from build123d import *

# Parameters (mm, degrees)
F2_R    = 2
F3_SIZE = 0.75


with BuildPart() as f1:
    # F0 (on Front) → F1 (revolve)
    with BuildSketch(Plane.XZ):
        Polygon((5.5, 0), (6.5, 30), (0, 30), (0, 15), (4, 15), (4, 0), align=None)
    revolve(axis=Axis((0, 0, 0.05881), (0, 0, -1)))

    # F2
    f2_edges = [f1.edges().sort_by_distance(p)[0] for p in [
        (-6.5, 0, 30),
    ]]
    fillet(f2_edges, radius=F2_R)

    # F3
    f3_edges = [f1.edges().sort_by_distance(p)[0] for p in [
        (-5.5, 0, 0),
    ]]
    chamfer(f3_edges, length=F3_SIZE)


solid = f1.part
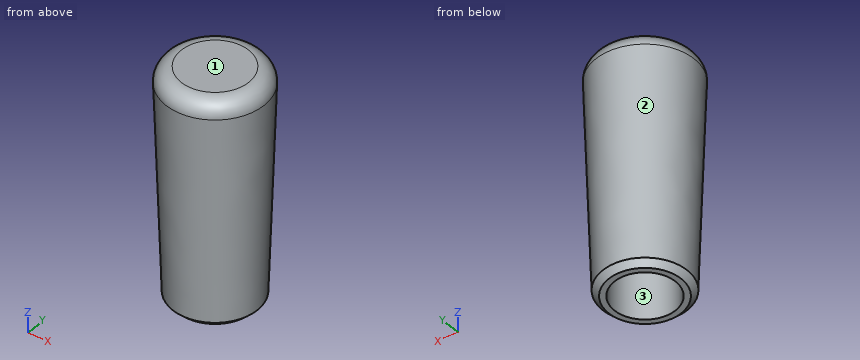
Verification items for the finished model (mm, model axes). Face numbers are marked on the shaded views. Round coordinates to 2 decimals unless told otherwise and drop trailing zeros. Loops run counter-clockwise (first coordinate to the right, second up) from the corner with the lowest first, then second, coordinate; pieces in that order, holes last. Notation, with made-up numbers: (86, -27.5) - (93, -27.5) arc R24 ccw to (93, 8.5) - close; hole circle Ø6 at (-6.75, 48). An arc over 180 degrees is marked (long way). Use one line per item in the form item = value.
1. Scan lines: probe 1 along X at (y, z) = (0, 10.5); probe 2 along X at (y, z) = (1, 13); probe 3 along Y at (x, z) = (1, 3). Record each from-to range of solid material in increasing order.
A:
probe_1 = -5.85 to -4, 4 to 5.85
probe_2 = -5.85 to -3.87, 3.87 to 5.85
probe_3 = -5.51 to -3.87, 3.87 to 5.51
2. Draft check along X on the marked faces 1, 2 and 3. Enter one of: pulls with the +X half, pulls with the -X half, needs draft (parallel to the pull), parting line crosses it, or undercut.
A:
face_1 = needs draft
face_2 = parting line crosses it
face_3 = undercut
3. Gauge pin test, flat ends, axial feed: pin 1 Ø6 at (x, z) = (2.5, 19) entering from -Y; pin 2 Ø2 at (x, y) = (0, -1.5) entering from -Z; pin 3 Ø1.5 at (x, z) = (5, 17.5) entering from -Y. Record the tip position at first contact, or that the pin passes through.
A:
pin_1 = -6.19
pin_2 = 15
pin_3 = -4.35
4. Section check C-C on z = 19.5. Record the cut outline in (x, y), and give its area (3 significant figures).
A:
outline = circle Ø12.3 at (0, 0)
area = 119 mm²
5. Section check A-A on y = 0. Record the cut outline in (x, z), and give its area (3 significant figures).
A:
outline = (-6.43, 27.93) - (-5.52, 0.75) - (-4.75, 0) - (-4, 0) - (-4, 15) - (4, 15) - (4, 0) - (4.75, 0) - (5.52, 0.75) - (6.43, 27.93) arc R2 ccw to (4.43, 30) - (-4.43, 30) arc R2 ccw to start
area = 238 mm²
